```python
from build123d import *

# Parameters (mm, degrees)
F1_DEPTH = 15
F2_DEPTH = 3
F3_R     = 1.65
F4_DEPTH = 5
F5_R     = 2.15
F6_DEPTH = 30


with BuildPart() as f1:
    # F0 (on Top) → F1 (new body)
    with BuildSketch(Plane.XY):
        Polygon((-53.4123483514, 9.8549427117), (-53.4123483514, 6.8549427117), (-16.4123483514, 6.8549427117), (-16.4123483514, 26.8549427117), (3.5876516486, 26.8549427117), (3.5876516486, 6.8549427117), (6.5876516486, 6.8549427117), (6.5876516486, 29.8549427117), (15.7216262448, 45.6754507873), (13.1235500334, 47.1754507873), (3.1235500334, 29.8549427117), (-1.0333719047, 32.2549427117), (8.9666280953, 49.5754507873), (6.3685518839, 51.0754507873), (-5.8831141659, 29.8549427117), (-19.4123483514, 29.8549427117), (-19.4123483514, 9.8549427117), align=None)
    extrude(amount=F1_DEPTH)

    # F0 (on Top) → F2 (join)
    with BuildSketch(Plane.XY):
        with BuildLine():
            add(Edge.make_bspline(
                [(-19.4123483514, 29.8549427117), (-25.070528026, 24.2659085839), (-35.6987359263, 13.7675822513), (-47.7683028951, 11.1016175788), (-53.4123483514, 9.8549427117)],
                knots=[0, 0, 0, 0, 0.5323738233, 1, 1, 1, 1], degree=3))
            Line((-53.4123483514, 9.8549427117), (-19.4123483514, 9.8549427117))
            Line((-19.4123483514, 9.8549427117), (-19.4123483514, 29.8549427117))
        make_face()
    extrude(amount=F2_DEPTH)

    # F3 (on face) → F4 (cut)
    with BuildSketch(Plane.XZ.offset(-6.8549427117)):
        with Locations((-48.4123483514, 9)):
            Circle(F3_R)
        with Locations((-24.5123483514, 9)):
            Circle(F3_R)
    extrude(amount=-F4_DEPTH, mode=Mode.SUBTRACT)

    # F5 (on face) → F6 (cut)
    with BuildSketch(Plane.YZ.offset(6.5876516486)):
        with Locations((16.8549427117, 7.5)):
            Circle(F5_R)
    extrude(amount=-F6_DEPTH, mode=Mode.SUBTRACT)


solid = f1.part
```
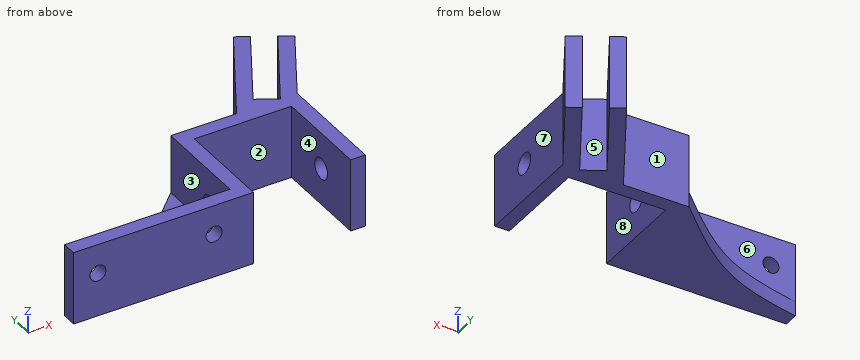
For this review, take the finished solid that the model builds, in its own axes (mm). Face numbers are marked on the shaded views. A direction names the side the tool comes from. Round coordinates to 2 decimals unless told otherwise and drop trailing zeros. Order: outer loops, then holes, each group sorted by start corner. A loop starts at its lowest first (then second) coordinate and runs counter-clockwise, first axis right, second up. Notation, with made-up numbers: (-0.5, -23.5) -> (31.5, -23.5) arc R17 cw to (31.5, -19.5) -> close; hole circle Ø1 at (52, 82.25). An arc over 180 degrees is marked (long way). Use a Markdown table: item, result.
Item 1: Take a section at C-C (x = -15). State the section outline as (y, z) points, plus the area to 3 significant figures.
Resolved:
| item | result |
|---|---|
| outline | (26.85, 0) -> (29.85, 0) -> (29.85, 15) -> (26.85, 15) -> close |
| area | 45.0 mm² |
Item 2: For line 1 along X through (y, z) = (16.5, 4); line 2 along Y through (x, z) = (5.5, 6.5); line 3 along Y through (x, z) = (-37, 7.5), list the stretches that pass through material, from the lowest coordinate up. Write a range as [from, to].
Resolved:
| item | result |
|---|---|
| line 1 | x = [-19.41, -16.41], [3.59, 6.59] |
| line 2 | y = [6.85, 14.95], [18.76, 33.97], [43.57, 49.57] |
| line 3 | y = [6.85, 9.85] |
Item 3: Take a section at A-A (z = 14). State the section outline as (x, y) points, plus the area to 3 significant figures.
Resolved:
| item | result |
|---|---|
| outline | (-53.41, 6.85) -> (-16.41, 6.85) -> (-16.41, 26.85) -> (3.59, 26.85) -> (3.59, 6.85) -> (6.59, 6.85) -> (6.59, 29.85) -> (15.72, 45.68) -> (13.12, 47.18) -> (3.12, 29.85) -> (-1.03, 32.25) -> (8.97, 49.58) -> (6.37, 51.08) -> (-5.88, 29.85) -> (-19.41, 29.85) -> (-19.41, 9.85) -> (-53.41, 9.85) -> close |
| area | 435 mm² |
Item 4: For pin 1 (8 mm diameter, centred on y = 45.5, z = 4.5, fed in from +X); pin 2 (4.5 mm diameter, centred on y = 13, z = 6, fed in from +X); pin 3 (3 mm diameter, centred on x = -40.5, z = 5, fed in from +Y); pin 4 (6 mm diameter, centred on x = -23, y = 25, fed in from -Z), all flat-tipped, find the tip position at first contact; note any pin that passes through.
Resolved:
| item | result |
|---|---|
| pin 1 | stops at x = 15.72 |
| pin 2 | stops at x = 6.59 |
| pin 3 | stops at y = 9.85 |
| pin 4 | stops at z = 0 |
Item 5: Take a section at B-B (y = 33.5). State the section outline as (x, z) points, plus the area to 3 significant figures.
Resolved:
| item | result |
|---|---|
| outline | (-3.78, 0) -> (-0.31, 0) -> (-0.31, 15) -> (-3.78, 15) -> close; (5.23, 0) -> (8.69, 0) -> (8.69, 15) -> (5.23, 15) -> close |
| area | 104 mm² |
Item 6: Draft analysis for pull direction X (two halves, no side actions). For the marked faces 1, 2, 3 and 4, state which applies: +X half, -X half, draft (parallel to the pull), parting line (faces both ways), or undercut.
Resolved:
| item | result |
|---|---|
| face 1 | draft |
| face 2 | undercut |
| face 3 | -X half |
| face 4 | undercut |
Item 7: Machinability: for the marked faces 5, 6, 7 and 8, which of the approach directions +Z, -Z, +X, -X, +Y, -Y give a long, thin tool a straight path to every point of the face, cutting with its end or side? Answer none if there is none.
Resolved:
| item | result |
|---|---|
| face 5 | +Z, -Z |
| face 6 | +Z, -X, +Y |
| face 7 | +Z, -Z, +X, -Y |
| face 8 | +Z, -Z, -Y |
Item 8: Take a section at D-D (x = -5). State the section outline as (y, z) points, plus the area to 3 significant figures.
Resolved:
| item | result |
|---|---|
| outline | (26.85, 0) -> (31.38, 0) -> (31.38, 15) -> (26.85, 15) -> close |
| area | 67.9 mm² |
